Geometry check sheet. Reference: the model listing, model coordinates, mm. A direction names the side the tool comes from. Give positions to 0.01 mm unless a question says otherwise; leave off trailing zeros. Loops run counter-clockwise (first coordinate to the right, second up) from the corner with the lowest first, then second, coordinate; pieces in that order, holes last. Notation, with made-up numbers: (8.25, 32.25) -> (15.25, 32.25) arc R32 ccw to (15.25, 63.25) -> close; hole circle Ø3 at (54, -28.5). An arc over 180 degrees is marked (long way). One line per question, with ' | ' between items.
Autodesk Inventor part; units mm, degrees
ref_plane "YZ Plane" through (0, 0, 0) normal (1, 0, 0) x (0, 1, 0)
ref_plane "XZ Plane" through (0, 0, 0) normal (0, 1, 0) x (-1, 0, 0)
ref_plane "XY Plane" through (0, 0, 0) normal (0, 0, 1) x (1, 0, 0)
sketch "Sketch1" plane through (0, 0, 0) normal (0, 1, 0) x (-1, 0, 0)
  circle A0 centre (0, 0) radius 2
  circle A1 centre (0, 0) radius 4 construction
  circle A2 centre (0, 0) radius 6.5
  dimension "d0" = 4
  dimension "d1" = 8
  dimension "d2" = 13
extrude "Extrusion1" add sketch "Sketch1" against normal blind 9
ref_plane "Work Plane1" through (0, -4.5, 0) normal (0, 1, 0) x (1, 0, 0)
hole "Hole1" at (0, 0, 0) direction (0, -1, 0) diameter 6 end through all counterbore diameter 8.2 counterbore depth 3
mirror "Mirror1" about plane through (0, -4.5, 0) normal (0, 1, 0) of "Hole1"
sketch "Sketch2" plane through (0, -4.5, 0) normal (0, 1, 0) x (1, 0, 0)
  circle A0 centre (0, 0) radius 4.1
  circle A1 centre (0, 0) radius 6.5
  line L0 (0, -6.5) -> (16.9987, -6.5)
  line L1 (16.9987, -6.5) -> (16.9987, 6.5)
  line L2 (16.9987, 6.5) -> (-0.0013, 6.5)
  arc A2 (-0.0013, 6.5) -> (0, -6.5) centre (0, 0) ccw
  dimension "d14" = 17
extrude "Extrusion2" add sketch "Sketch2" against normal up to surface (9 mm away) from surface at 4.5 contours A1 L2 L1 L0
sketch "Sketch3" plane through (16.9987, -9, -6.5) normal (1, 0, 0) x (0, 0, -1)
  line L0 (-13, 0) -> (-13, 9) construction
  line L1 (-13, 4.5) -> (0, 4.5) construction
  line L2 (0, 0) -> (0, 9) construction
  line L3 (-6.5, 9) -> (-6.5, -1) construction
  line L4 (-12, 6.5) -> (-1, 6.5)
  line L5 (-1, 6.5) -> (-1, 2.5)
  line L6 (-1, 2.5) -> (-12, 2.5)
  line L7 (-12, 2.5) -> (-12, 6.5)
  dimension "d17" = 11
  dimension "d18" = 4
extrude "Extrusion3" cut sketch "Sketch3" against normal blind 10
sketch "Sketch4" plane through (0, -4.5, 0) normal (0, 1, 0) x (1, 0, 0)
  line L0 (16.9987, 6.5) -> (16.9987, -6.5)
  line L1 (16.9987, -6.5) -> (4.9987, -6.5)
  line L2 (4.9987, -6.5) -> (4.9987, -7.5)
  line L3 (4.9987, -7.5) -> (16.9987, -7.5)
  line L4 (16.9987, -7.5) -> (16.9987, -6.5)
  line L5 (0, 0) -> (21.5191, 0) construction
  line L6 (16.9987, 6.5) -> (4.9987, 6.5)
  line L7 (4.9987, 6.5) -> (4.9987, 7.5)
  line L8 (4.9987, 7.5) -> (16.9987, 7.5)
  line L9 (16.9987, 7.5) -> (16.9987, 6.5)
  dimension "d21" = 1
  dimension "d22" = 12
extrude "Extrusion4" add sketch "Sketch4" against normal up to surface (9 mm away) from surface at 4.5
fillet "Fillet1" radius 2 2 edges at (4.9987, -4.5, -6.5) (4.9987, -4.5, 6.5)
sketch "Sketch5" plane through (0, -4.5, 0) normal (0, 1, 0) x (1, 0, 0)
  line L0 (16.9987, -5.5) -> (6.9987, -5.5) construction
  line L1 (6.9987, -5.5) -> (6.9987, 5.5) construction
  line L2 (16.9987, 5.5) -> (6.9987, 5.5) construction
  line L3 (6.9987, 0) -> (20.6867, 0) construction
  line L4 (11.9987, -5.5) -> (11.9987, 4.4002) construction
  circle A0 centre (11.9987, 0) radius 1.75
  point P0 (0, 0)
  dimension "d26" = 3.5
extrude "Extrusion5" cut sketch "Sketch5" along normal through all both and the other way through all
properties part number "center-machine-v2-rod-socket"
Item 1: Scan lines: probe 1 along Z at (x, y) = (12.5, -6); probe 2 along X at (y, z) = (-3.85, 0); probe 3 along X at (y, z) = (-8.5, 0.25). Record each from-to range of solid material in increasing order.
Result:
probe 1: -7.5 to -5.5, 5.5 to 7.5 | probe 2: -6.5 to -3, 3 to 7 | probe 3: -6.5 to -4.09, 4.09 to 10.27, 13.73 to 17
Item 2: Set-up check for faces 1 (the face through (1, -3, -3)), 2 (the face through (2, -4, -6.5)), 3 (the face through (2, -4, 6.5)), 4 (the face through (10.25, -1.27, 0.08)), 5 (the face through (6.999, -4, 0)): record each of +Z, -Z, +X, -X, +Y, -Y from which the full face is reachable in a straight line by a thin tool's end or side.
Result:
face 1: +Y | face 2: -Z, -X, +Y, -Y | face 3: +Z, -X, +Y, -Y | face 4: +Y, -Y | face 5: +X
Item 3: Release check for a two-part mould opening along Y. For faces 6 (the face through (1, -6, 3)), 7 (the face through (12, -4, -5.5)), 8 (the face through (10.25, -7.73, -0.08)) record: pulls with the +Y half, pulls with the -Y half, needs draft (parallel to the pull), parting line crosses it, or undercut.
Result:
face 6: pulls with the -Y half | face 7: undercut | face 8: needs draft
Item 4: Depth check by flat-ended pin: pin 1 Ø8 at (x, z) = (0, 0) entering from +Y; pin 2 Ø5 at (x, z) = (0, 0) entering from +Y; pin 3 Ø2.5 at (x, z) = (0.5, -2) entering from -Y; pin 4 Ø1.5 at (x, y) = (-0.5, -4.5) entering from +Z. Enter the tip coordinate at first touch or a pass-through.
Result:
pin 1: y = -3 | pin 2: through | pin 3: y = -6 | pin 4: z = 6.5
Item 5: Sectioned sample at B-B (x = 0.75). Record the cut outline in (y, z).
Result:
outline: (-9, -6.5) -> (0, -6.5) -> (0, -4.03) -> (-3, -4.03) -> (-3, -2.9) -> (-6, -2.9) -> (-6, -4.03) -> (-9, -4.03) -> close; (-9, 4.03) -> (-6, 4.03) -> (-6, 2.9) -> (-3, 2.9) -> (-3, 4.03) -> (0, 4.03) -> (0, 6.5) -> (-9, 6.5) -> close
Item 6: Sectioned sample at D-D (x = 9). Record the cut outline in (y, z), plus the area to 3 significant figures.
Result:
outline: (-9, -7.5) -> (0, -7.5) -> (0, 7.5) -> (-9, 7.5) -> close; hole (-6.5, -5.5) -> (-2.5, -5.5) -> (-2.5, 5.5) -> (-6.5, 5.5) -> close | area: 91.0 mm2
Item 7: Sectioned sample at A-A (z = 0). Record the cut outline in (x, y), plus the area to 3 significant figures.
Result:
outline: (-6.5, -9) -> (-4.1, -9) -> (-4.1, -6) -> (-3, -6) -> (-3, -3) -> (-4.1, -3) -> (-4.1, 0) -> (-6.5, 0) -> close; (3, -6) -> (4.1, -6) -> (4.1, -9) -> (10.25, -9) -> (10.25, -6.5) -> (7, -6.5) -> (7, -2.5) -> (10.25, -2.5) -> (10.25, 0) -> (4.1, 0) -> (4.1, -3) -> (3, -3) -> close; (13.75, -9) -> (17, -9) -> (17, -6.5) -> (13.75, -6.5) -> close; (13.75, -2.5) -> (17, -2.5) -> (17, 0) -> (13.75, 0) -> close | area: 86.8 mm2
Item 8: Sectioned sample at C-C (y = -3.5). Record the cut outline in (x, z), plus the area to 3 significant figures.
Result:
outline: (0, -6.5) -> (3.27, -6.5) arc R2 cw to (5, -7.5) -> (17, -7.5) -> (17, -5.5) -> (7, -5.5) -> (7, 5.5) -> (17, 5.5) -> (17, 7.5) -> (5, 7.5) arc R2 cw to (3.27, 6.5) -> (0, 6.5) arc R6.5 ccw to start; hole circle Ø6 at (0, 0) | area: 174 mm2
